Design review of the part built by this model. Coordinates are the model's own, in mm. Face numbers are marked on the shaded views. A direction names the side the tool comes from. Coordinates: 2 decimals unless noted, no trailing zeros. Loops run counter-clockwise (first coordinate to the right, second up) from the corner with the lowest first, then second, coordinate; pieces in that order, holes last.
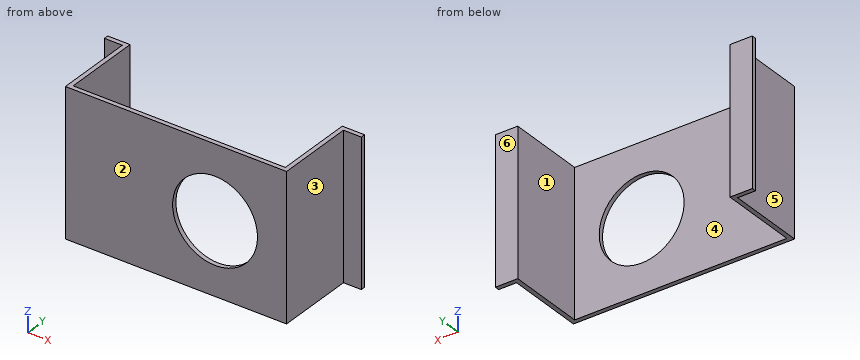
from build123d import *

# Parameters (mm, degrees)
BOSS_EXTRUDE1_DEPTH = 65
SKETCH2_R           = 19
CUT_EXTRUDE1_DEPTH  = 125.693619771


with BuildPart() as part:
    # Sketch1 → Boss-Extrude1 (new body)
    with BuildSketch(Plane.XY):
        Polygon((-15.227765327, 6.012341763), (-5.227765327, 6.012341763), (-5.227765327, -28.987658237), (89.772234673, -28.987658237), (89.772234673, 6.012341763), (99.772234673, 6.012341763), (99.772234673, 4.012341763), (91.772234673, 4.012341763), (91.772234673, -30.987658237), (-7.227765327, -30.987658237), (-7.227765327, 4.012341763), (-15.227765327, 4.012341763), align=None)
    extrude(amount=BOSS_EXTRUDE1_DEPTH)

    # Sketch2 → Cut-Extrude1 (cut, through all)
    with BuildSketch(Plane.XZ.offset(30.987658237)):
        with Locations((59.772234673, 32.253053016)):
            Circle(SKETCH2_R)
    extrude(amount=-CUT_EXTRUDE1_DEPTH, mode=Mode.SUBTRACT)


solid = part.part
Q1. Take a section at A-A, the plane y = -23.5. Write out the cut boundary in (x, z), then the cut area to 3 significant figures.
Q2. Clearance check with flat-ended pins moving along their axes: pin 1 Ø6 at (x, y) = (32, -23.5) entering from +Z; pin 2 Ø6 at (y, z) = (-2.5, 40) entering from -X; pin 3 Ø10 at (x, z) = (72, 56) entering from +Y; pin 4 Ø4 at (x, z) = (97, 30) entering from -Y. State where each tip first meets the part, or that it passes through.
Q3. Take a section at C-C, the plane x = 59. Write out the cut boundary in (y, z), then the cut area to 3 significant figures.
Q4. Take a section at B-B, the plane z = 54. Write out the cut boundary in (x, y).
Q5. For line 1 (X direction, y = -0.5, z = 22.5); line 2 (Y direction, x = 89, z = 28), list the stretches that pass through material, from the lowest coordinate up.
Q6. Take a section at D-D, the plane z = 29. Write out the cut boundary in (x, y).
Q7. The part is to be moulded in two halves that separate along X. For the marked faces 4, 5 and 6, say which applies: pulls with the +X half, pulls with the -X half, needs draft (parallel to the pull), parting line crosses it, or undercut.
Q8. Machinability: for the marked faces 1, 2 and 3, which of the approach directions +Z, -Z, +X, -X, +Y, -Y give a long, thin tool a straight path to every point of the face, cutting with its end or side? Answer none if there is none.
Entries:
1. outline: (-7.23, 0) - (-5.23, 0) - (-5.23, 65) - (-7.23, 65) - close; (89.77, 0) - (91.77, 0) - (91.77, 65) - (89.77, 65) - close
1. area: 260 mm2
2. pin 1: passes through
2. pin 2: stops at x = -7.23
2. pin 3: stops at y = -28.99
2. pin 4: stops at y = 4.01
3. outline: (-30.99, 0) - (-28.99, 0) - (-28.99, 13.27) - (-30.99, 13.27) - close; (-30.99, 51.24) - (-28.99, 51.24) - (-28.99, 65) - (-30.99, 65) - close
3. area: 54.1 mm2
4. outline: (-15.23, 4.01) - (-7.23, 4.01) - (-7.23, -30.99) - (91.77, -30.99) - (91.77, 4.01) - (99.77, 4.01) - (99.77, 6.01) - (89.77, 6.01) - (89.77, -28.99) - (-5.23, -28.99) - (-5.23, 6.01) - (-15.23, 6.01) - close
5. line 1: x = -7.23 to -5.23, 89.77 to 91.77
5. line 2: y = -30.99 to -28.99
6. outline: (-15.23, 4.01) - (-7.23, 4.01) - (-7.23, -30.99) - (41.05, -30.99) - (41.05, -28.99) - (-5.23, -28.99) - (-5.23, 6.01) - (-15.23, 6.01) - close; (78.49, -30.99) - (91.77, -30.99) - (91.77, 4.01) - (99.77, 4.01) - (99.77, 6.01) - (89.77, 6.01) - (89.77, -28.99) - (78.49, -28.99) - close
7. face 4: undercut
7. face 5: pulls with the -X half
7. face 6: needs draft
8. face 1: +Z, -Z, +Y
8. face 2: +Z, -Z, +X, -X, -Y
8. face 3: +Z, -Z, +X, -Y
